```python
from build123d import *

# Parameters (mm, degrees)
SKETCH_1_W               = 200
SKETCH_1_H               = 206
EXTRUDE_2_DEPTH          = 5
SKETCH_2_W               = 200
SKETCH_2_H               = 8
EXTRUDE_3_DEPTH          = 70
SKETCH_3_W               = 5
SKETCH_3_H               = 190
EXTRUDE_4_DEPTH          = 54.7
SKETCH_4_W               = 200
SKETCH_4_H               = 8
EXTRUDE_5_DEPTH          = 70
SKETCH_14_W              = 5
SKETCH_14_H              = 190
EXTRUDE_7_DEPTH          = 65.3
SKETCH_15_W              = 5
SKETCH_15_H              = 50
CUT_EXTRUDE_7_DEPTH      = 3
CUT_EXTRUDE_8_DEPTH      = 1
CUT_EXTRUDE_8_DEPTH_BACK = 8
CUT_EXTRUDE_9_DEPTH      = 1
CUT_EXTRUDE_9_DEPTH_BACK = 8
SKETCH_19_R              = 1.5
CUT_EXTRUDE_10_DEPTH     = 5
SKETCH_21_W              = 30
SKETCH_21_H              = 8
EXTRUDE_8_DEPTH          = 10
SKETCH_24_W              = 5
SKETCH_24_H              = 6.5
CUT_EXTRUDE_11_DEPTH     = 196
SKETCH_25_W              = 2.5
SKETCH_25_H              = 3.5
CUT_EXTRUDE_12_DEPTH     = 196
CUT_EXTRUDE_13_DEPTH     = 196
SKETCH_27_W              = 5
SKETCH_27_H              = 6.5
CUT_EXTRUDE_14_DEPTH     = 196
SKETCH_28_W              = 2.5
SKETCH_28_H              = 3.467533866
CUT_EXTRUDE_15_DEPTH     = 196
CUT_EXTRUDE_16_DEPTH     = 196


with BuildPart() as part:
    # Эскиз1 → Бобышка-Вытянуть2 (new body)
    with BuildSketch(Plane(origin=(0, 0, 0), x_dir=(1, 0, 0), z_dir=(0, 1, 0))):
        Rectangle(SKETCH_1_W, SKETCH_1_H)
    extrude(amount=EXTRUDE_2_DEPTH)

    # Эскиз2 → Бобышка-Вытянуть3 (add)
    with BuildSketch(Plane(origin=(0, 5, 0), x_dir=(1, 0, 0), z_dir=(0, 1, 0))):
        with Locations((0, -99)):
            Rectangle(SKETCH_2_W, SKETCH_2_H)
    extrude(amount=EXTRUDE_3_DEPTH)

    # Эскиз3 → Бобышка-Вытянуть4 (add)
    with BuildSketch(Plane(origin=(0, 5, 0), x_dir=(1, 0, 0), z_dir=(0, 1, 0))):
        with Locations((97.5, 0)):
            Rectangle(SKETCH_3_W, SKETCH_3_H)
    extrude(amount=EXTRUDE_4_DEPTH)

    # Эскиз4 → Бобышка-Вытянуть5 (add)
    with BuildSketch(Plane(origin=(0, 5, 0), x_dir=(1, 0, 0), z_dir=(0, 1, 0))):
        with Locations((0, 99)):
            Rectangle(SKETCH_4_W, SKETCH_4_H)
    extrude(amount=EXTRUDE_5_DEPTH)

    # Эскиз14 → Бобышка-Вытянуть7 (add)
    with BuildSketch(Plane(origin=(0, 5, 0), x_dir=(1, 0, 0), z_dir=(0, 1, 0))):
        with Locations((-97.5, 0)):
            Rectangle(SKETCH_14_W, SKETCH_14_H)
    extrude(amount=EXTRUDE_7_DEPTH)

    # Эскиз15 → Вырез-Вытянуть7 (cut)
    with BuildSketch(Plane(origin=(0, 70.3, 0), x_dir=(1, 0, 0), z_dir=(0, 1, 0))):
        with Locations((-97.5, 0)):
            Rectangle(SKETCH_15_W, SKETCH_15_H)
    extrude(amount=-CUT_EXTRUDE_7_DEPTH, mode=Mode.SUBTRACT)

    # Эскиз16 → Вырез-Вытянуть8 (cut, two sides)
    with BuildSketch(Plane(origin=(0, 0, -103), x_dir=(-1, 0, 0), z_dir=(0, 0, -1))) as cut_extrude_8_sk:
        with BuildLine():
            Line((-19, 366.325434328), (-19, 75))
            ThreePointArc((-19, 75), (-18, 74), (-17, 75))
            Line((-17, 75), (-17, 366.325434328))
            Line((-17, 366.325434328), (-17, 948.976302985))
            Line((-17, 948.976302985), (-19, 948.976302985))
            Line((-19, 948.976302985), (-19, 366.325434328))
        make_face()
    extrude(amount=CUT_EXTRUDE_8_DEPTH, mode=Mode.SUBTRACT)
    extrude(cut_extrude_8_sk.sketch, amount=-CUT_EXTRUDE_8_DEPTH_BACK, mode=Mode.SUBTRACT)

    # Эскиз18 → Вырез-Вытянуть9 (cut, two sides)
    with BuildSketch(Plane(origin=(0, 0, -103), x_dir=(-1, 0, 0), z_dir=(0, 0, -1))) as cut_extrude_9_sk:
        with BuildLine():
            Line((17, 366.325434328), (17, 75))
            ThreePointArc((17, 75), (18, 74), (19, 75))
            Line((19, 75), (19, 366.325434328))
            Line((19, 366.325434328), (19, 948.976302985))
            Line((19, 948.976302985), (17, 948.976302985))
            Line((17, 948.976302985), (17, 366.325434328))
        make_face()
    extrude(amount=CUT_EXTRUDE_9_DEPTH, mode=Mode.SUBTRACT)
    extrude(cut_extrude_9_sk.sketch, amount=-CUT_EXTRUDE_9_DEPTH_BACK, mode=Mode.SUBTRACT)

    # Эскиз19 → Вырез-Вытянуть10 (cut)
    with BuildSketch(Plane(origin=(0, 0, -103), x_dir=(-1, 0, 0), z_dir=(0, 0, -1))):
        with Locations((0, 70)):
            Circle(SKETCH_19_R)
    extrude(amount=-CUT_EXTRUDE_10_DEPTH, mode=Mode.SUBTRACT)

    # Эскиз21 → Бобышка-Вытянуть8 (add)
    with BuildSketch(Plane(origin=(0, 75, 0), x_dir=(1, 0, 0), z_dir=(0, 1, 0))):
        with Locations((-80, -99)):
            Rectangle(SKETCH_21_W, SKETCH_21_H)
        with Locations((-40, -99)):
            Rectangle(SKETCH_21_W, SKETCH_21_H)
        with Locations((0, -99)):
            Rectangle(SKETCH_21_W, SKETCH_21_H)
        with Locations((40, -99)):
            Rectangle(SKETCH_21_W, SKETCH_21_H)
        with Locations((80, -99)):
            Rectangle(SKETCH_21_W, SKETCH_21_H)
        with Locations((80, 99)):
            Rectangle(SKETCH_21_W, SKETCH_21_H)
        with Locations((40, 99)):
            Rectangle(SKETCH_21_W, SKETCH_21_H)
        with Locations((-40, 99)):
            Rectangle(SKETCH_21_W, SKETCH_21_H)
        with Locations((-80, 99)):
            Rectangle(SKETCH_21_W, SKETCH_21_H)
    extrude(amount=EXTRUDE_8_DEPTH)

    # Эскиз24 → Вырез-Вытянуть11 (cut, through all)
    with BuildSketch(Plane(origin=(95, 0, 0), x_dir=(0, 0, -1), z_dir=(1, 0, 0))):
        with Locations((-97.5, 78.25)):
            Rectangle(SKETCH_24_W, SKETCH_24_H)
    extrude(amount=-CUT_EXTRUDE_11_DEPTH, mode=Mode.SUBTRACT)

    # Эскиз25 → Вырез-Вытянуть12 (cut, through all)
    with BuildSketch(Plane(origin=(95, 0, 0), x_dir=(0, 0, -1), z_dir=(1, 0, 0))):
        with Locations((-96.25, 83.25)):
            Rectangle(SKETCH_25_W, SKETCH_25_H)
    extrude(amount=-CUT_EXTRUDE_12_DEPTH, mode=Mode.SUBTRACT)

    # Эскиз26 → Вырез-Вытянуть13 (cut, through all)
    with BuildSketch(Plane(origin=(95, 0, 0), x_dir=(0, 0, -1), z_dir=(1, 0, 0))):
        Polygon((-97.5, 81.5), (-100.25, 85), (-97.5, 85), align=None)
    extrude(amount=-CUT_EXTRUDE_13_DEPTH, mode=Mode.SUBTRACT)

    # Эскиз27 → Вырез-Вытянуть14 (cut, through all)
    with BuildSketch(Plane(origin=(95, 0, 0), x_dir=(0, 0, -1), z_dir=(1, 0, 0))):
        with Locations((97.5, 78.282466134)):
            Rectangle(SKETCH_27_W, SKETCH_27_H)
    extrude(amount=-CUT_EXTRUDE_14_DEPTH, mode=Mode.SUBTRACT)

    # Эскиз28 → Вырез-Вытянуть15 (cut, through all)
    with BuildSketch(Plane(origin=(95, 0, 0), x_dir=(0, 0, -1), z_dir=(1, 0, 0))):
        with Locations((96.25, 83.266233067)):
            Rectangle(SKETCH_28_W, SKETCH_28_H)
    extrude(amount=-CUT_EXTRUDE_15_DEPTH, mode=Mode.SUBTRACT)

    # Эскиз29 → Вырез-Вытянуть16 (cut, through all)
    with BuildSketch(Plane(origin=(95, 0, 0), x_dir=(0, 0, -1), z_dir=(1, 0, 0))):
        Polygon((97.5, 81.532466134), (100.25, 85), (97.5, 85), align=None)
    extrude(amount=-CUT_EXTRUDE_16_DEPTH, mode=Mode.SUBTRACT)


solid = part.part
```
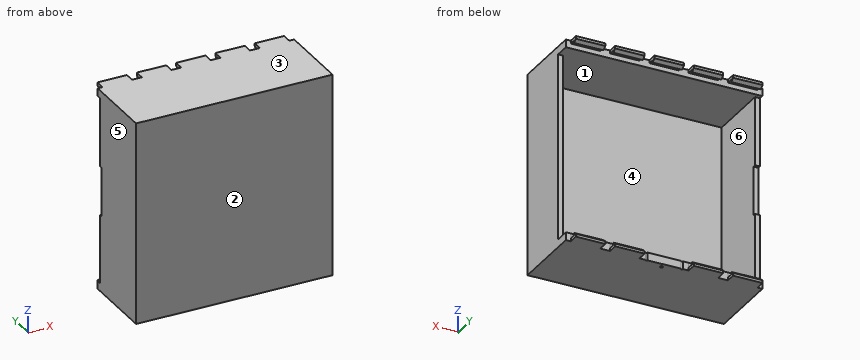
Source: CAD feature listing. Evaluate the final solid. Frame: model axes, mm. Face numbers are marked on the shaded views. A direction names the side the tool comes from. Coordinates: 2 decimals unless noted, no trailing zeros. Loops run counter-clockwise (first coordinate to the right, second up) from the corner with the lowest first, then second, coordinate; pieces in that order, holes last. Notation, with made-up numbers: (58, -26.75) -> (92, -26.75) arc R35 ccw to (92, 8.25) -> close; hole circle Ø3 at (55, -33.75). An arc over 180 degrees is marked (long way). One line per item, written item: value. Start each with the question number.
Q1. Mould query, pull axis Z, two halves, no side actions, for the marked faces 3, 4, 5 and 6. Classes: pulls with the +Z half, pulls with the -Z half, needs draft (parallel to the pull), parting line crosses it, or undercut.
Q2. Contact query for flat-ended pins moving along their axis: P1, Ø4, axis at x = 98.5, z = 26.5, coming from the +Y side; P2, Ø3, axis at y = 79.5, z = 100.5, coming from the -X side; P3, Ø1, axis at y = 72.5, z = 32, coming from the +X side; P4, Ø3, axis at x = -8.5, z = -37, coming from the +Y side. Output: stop coordinate, or through.
Q3. Section query D-D, the plane x = -81. Return the cut outline in (y, z), and give its area (3 significant figures).
Q4. Line query: line 1 along Y through (x, z) = (0, -101.8); line 2 along Z through (x, y) = (78.5, 77); line 3 along Z through (x, y) = (73, 15). Output: solid intervals per line, ascending.
Q5. Section query A-A, the plane z = 63. Return the cut outline in (x, y), and give its area (3 significant figures).
Q6. Set-up query: the marked faces 1 and 2. Return all of +Z, -Z, +X, -X, +Y, -Y with unobstructed straight access to the full face (end or side cutting, diameter ignored); none if empty.
Q7. Section query B-B, the plane y = 49. Return the cut outline in (x, z).
Q8. Section query C-C, the plane x = 22. Return the cut outline in (y, z).
Results:
1. face 3: pulls with the +Z half
1. face 4: undercut
1. face 5: needs draft
1. face 6: undercut
2. P1: y = 59.7
2. P2: x = -95
2. P3: through
2. P4: y = 5
3. outline: (0, -103) -> (85, -103) -> (85, -100.25) -> (81.53, -97.5) -> (81.53, -100) -> (75.03, -100) -> (75.03, -95) -> (5, -95) -> (5, 95) -> (75, 95) -> (75, 100) -> (81.5, 100) -> (81.5, 97.5) -> (85, 100.25) -> (85, 103) -> (0, 103) -> close
3. area: 2,220 mm^2
4. line 1: 0 to 68.5, 71.5 to 75
4. line 2: -103 to -100, 100 to 103
4. line 3: -103 to -95, 95 to 103
5. outline: (-100, 0) -> (100, 0) -> (100, 59.7) -> (95, 59.7) -> (95, 5) -> (-95, 5) -> (-95, 70.3) -> (-100, 70.3) -> close
5. area: 1,600 mm^2
6. face 1: +Y
6. face 2: +Z, -Z, +X, -X, -Y
7. outline: (-100, -103) -> (100, -103) -> (100, 103) -> (-100, 103) -> close; hole (-95, -95) -> (95, -95) -> (95, 95) -> (-95, 95) -> close
8. outline: (0, -103) -> (75, -103) -> (75, -95) -> (5, -95) -> (5, 95) -> (75, 95) -> (75, 103) -> (0, 103) -> close
